Can you work these out from the model? Positions are in its coordinate system, mm. A direction names the side the tool comes from. Round coordinates to 2 decimals unless told otherwise and drop trailing zeros. Order: outer loops, then holes, each group sorted by start corner. A loop starts at its lowest first (then second) coordinate and runs counter-clockwise, first axis right, second up. Notation, with made-up numbers: (71, -28.5) -> (106, -28.5) arc R23 ccw to (106, 1.5) -> close; hole circle Ø1 at (-11.75, 23.5). An arc over 180 degrees is marked (long way). Use a Markdown table: item, result. Add a question column.
Q1. If we section it at D-D on y = -10: List the corners of the cut face in (x, z) for me.
Q2. I'm going to push flat-ended pins straight in: pin 1 Ø2 at (x, y) = (7, 24) entering from +Z; pin 2 Ø3 at (x, z) = (-11.5, 2.5) entering from +Y; pin 3 Ø1.5 at (y, z) = (41, -8) entering from +X. Where does each tip first touch, or does it pass through?
Q3. For faces 1 (the face through (0, -25, 0)), 2 (the face through (-4, 44, 3)), 3 (the face through (10, 23.93, 0)), which set-ups out of +Z, -Z, +X, -X, +Y, -Y let a thin tool reach every point of the face, with its end or its side?
Q4. If we section it at B-B on z = 2.75: List the corners of the cut face in (x, y) for me, plus the area to 3 significant figures.
Q5. If we section it at A-A on y = 49: List the corners of the cut face in (x, z) for me.
Q6. If we section it at C-C on x = 0: List the corners of the cut face in (y, z) for me, plus the area to 3 significant figures.
Q7. I need wall thicknesses on line 1 along X through (y, z) = (33, 8.5); line 2 along Z through (x, y) = (2.75, 50); line 3 along Z through (x, y) = (-3.75, 28.5). Which ranges of each line are inside material? Lowest first, please. Write a range as [from, to].
Q8. We'd pull the mould along Z, two halves only. Please class faces 4 (the face through (-0.204, 51.224, 0.258)), 5 (the face through (0.55, 5.551, -12.488)), 6 (the face through (-5.43, 25.43, 0.17)): +Z half, -Z half, draft (parallel to the pull), parting line (faces both ways), or undercut.
```python
from build123d import *

# Parameters (mm, degrees)
EXTRUDE_START       = -25
SKETCH_1_R          = 12.5
EXTRUDE_1_DEPTH     = 85
SKETCH_2_W          = 12.354431351
SKETCH_2_H          = 42
SKETCH_2_W_2        = 12.054431351
CUT_EXTRUDE_2_DEPTH = 30
FILLET_2_R          = 5
SKETCH_3_R          = 4
CUT_EXTRUDE_1_DEPTH = 64.470465687
FILLET_3_R          = 5


with BuildPart() as part:
    # Эскиз1 → Вытянуть1 (new body)
    with BuildSketch(Plane(origin=(0, 0, 0), x_dir=(1, 0, 0), z_dir=(0, 1, 0)).offset(EXTRUDE_START)):
        with Locations(Location((0, 0, 0), (0, 0, 270))):
            Circle(SKETCH_1_R)
    extrude(amount=EXTRUDE_1_DEPTH)

    # Эскиз2 → Вытянуть2 (cut, symmetric)
    with BuildSketch(Plane.XY):
        with Locations((9.877215676, 44.929871577)):
            Rectangle(SKETCH_2_W, SKETCH_2_H)
        with Locations((-10.027215676, 44.929871577)):
            Rectangle(SKETCH_2_W_2, SKETCH_2_H)
    extrude(amount=CUT_EXTRUDE_2_DEPTH, both=True, mode=Mode.SUBTRACT)

    # Скругление2
    fillet_2_edges = [part.edges().sort_by_distance(p)[0] for p in [
        (-0.157665968, 60, -12.499005618),
        (-2.026821276, 60, 12.33458534),
    ]]
    fillet(fillet_2_edges, radius=FILLET_2_R)

    # Эскиз3 → Вырез-Вытянуть1 (cut, through all)
    with BuildSketch(Plane.ZY.offset(4)):
        with Locations(Location((0.082516108, 47.227633341, 0), (0, 0, 270))):
            Circle(SKETCH_3_R)
    extrude(amount=-CUT_EXTRUDE_1_DEPTH, mode=Mode.SUBTRACT)

    # Скругление3
    fillet_3_edges = [part.edges().sort_by_distance(p)[0] for p in [
        (3.7, 23.929871577, 0),
        (-4, 23.929871577, 0),
    ]]
    fillet(fillet_3_edges, radius=FILLET_3_R)


solid = part.part
```
Answer below:
| question | item | result |
|---|---|---|
| 1 | outline | circle Ø25 at (0, 0) |
| 2 | pin 1 | z = 10.97 |
| 2 | pin 2 | y = 23.93 |
| 2 | pin 3 | x = 3.7 |
| 3 | face 1 | +Z, -Z, +X, -X, -Y |
| 3 | face 2 | +Z, -Z, -X, +Y |
| 3 | face 3 | +Z, -Z, +X, +Y |
| 4 | outline | (-12.19, -25) -> (12.19, -25) -> (12.19, 23.93) -> (8.7, 23.93) arc R5 cw to (3.7, 28.93) -> (3.7, 44.25) -> (-4, 44.25) -> (-4, 28.93) arc R5 cw to (-9, 23.93) -> (-12.19, 23.93) -> close; (-4, 50.21) -> (3.7, 50.21) -> (3.7, 60) -> (-4, 60) -> close |
| 4 | area | 1,440 mm² |
| 5 | outline | (-4, -11.84) arc R12.5 ccw to (3.7, -11.94) -> (3.7, -3.5) -> (-4, -3.5) -> close; (-4, 3.67) -> (3.7, 3.67) -> (3.7, 11.94) arc R12.5 ccw to (-4, 11.84) -> close |
| 6 | outline | (-25, -12.5) -> (55, -12.5) arc R5 ccw to (60, -7.5) -> (60, 7.5) arc R5 ccw to (55, 12.5) -> (-25, 12.5) -> close; hole circle Ø8 at (47.23, 0.08) |
| 6 | area | 2,060 mm² |
| 7 | line 1 | [-4, 3.7] |
| 7 | line 2 | [-12.19, -2.8], [2.97, 12.19] |
| 7 | line 3 | [-11.92, 11.92] |
| 8 | face 4 | undercut |
| 8 | face 5 | parting line |
| 8 | face 6 | draft |
